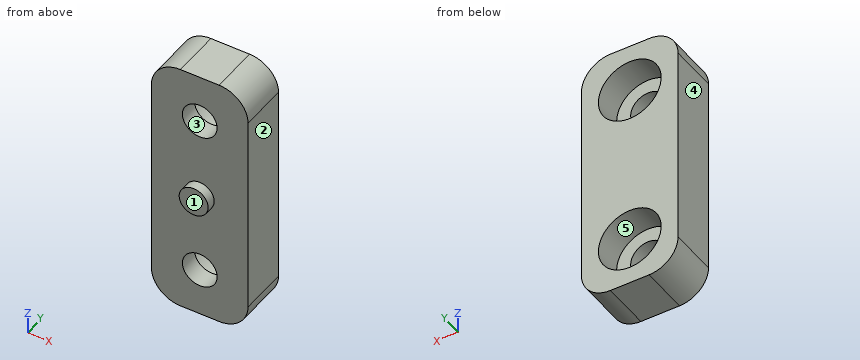
Autodesk Inventor part; units mm, degrees
ref_plane "YZ Plane" through (0, 0, 0) normal (1, 0, 0) x (0, 1, 0)
ref_plane "XZ Plane" through (0, 0, 0) normal (0, 1, 0) x (-1, 0, 0)
ref_plane "XY Plane" through (0, 0, 0) normal (0, 0, 1) x (1, 0, 0)
sketch "Sketch1" plane through (0, 0, 0) normal (0, 1, 0) x (-1, 0, 0)
  line L0 (5, -13.5) -> (-5, -13.5)
  line L1 (-5, -13.5) -> (-5, 13.5)
  line L2 (-5, 13.5) -> (5, 13.5)
  line L3 (5, 13.5) -> (5, -13.5)
  line L4 (5, -13.5) -> (-5, 13.5) construction
  line L5 (-5, -13.5) -> (5, 13.5) construction
  circle A0 centre (0, -8.5) radius 3.25
  circle A1 centre (0, 8.5) radius 3.25
  circle A2 centre (0, 0) radius 1.5
  dimension "d0" = 17
  dimension "d1" = 6.5
  dimension "d2" = 6.5
  dimension "d3" = 3
  dimension "d4" = 5
  dimension "d5" = 5
  dimension "d6" = 5
extrude "Extrusion1" add sketch "Sketch1" along normal blind 5 contours L0 L1 L2 L3 | A0 | A1 | A2
sketch "Sketch2" plane through (0, 0, 0) normal (0, -1, 0) x (1, 0, 0)
  circle A0 centre (0, 0) radius 1.5
  dimension "d9" = 3
extrude "Extrusion2" add sketch "Sketch2" along normal blind 1
sketch "Sketch3" plane through (0, 5, 0) normal (0, 1, 0) x (1, 0, 0)
  line L0 (-5, -13.5) -> (5, -13.5)
  line L1 (5, -13.5) -> (5, 13.5)
  line L2 (5, 13.5) -> (-5, 13.5)
  line L3 (-5, 13.5) -> (-5, -13.5)
  point P0 (0, 0)
  point P1 (0, 8.5)
  point P2 (0, -8.5)
  dimension "d12" = 8.5
  dimension "d13" = 8.5
hole "Hole1" at (0, 5, -8.5) at (0, 5, 8.5) direction (0, -1, 0) diameter 3.6 depth 28.25 tip angle 118 counterbore diameter 6.5 counterbore depth 3
fillet "Fillet1" radius 3 4 edges at (5, 2.5, 13.5) (5, 2.5, -13.5) (-5, 2.5, -13.5) (-5, 2.5, 13.5)
sketch "Sketch4" plane through (0, 2, -8.5) normal (0, 1, 0) x (1, 0, 0)
  circle A0 centre (0, 0) radius 1.8
  circle A1 centre (0, -17) radius 1.8
  point P0 (0, -8.5)
extrude "Extrusion3" [suppressed]
properties part number "Belt Clamp Block" material "ABS Plastic"
Design review of the part built by this model. Coordinates are the model's own, in mm. Face numbers are marked on the shaded views. A direction names the side the tool comes from. Coordinates: 2 decimals unless noted, no trailing zeros. Loops run counter-clockwise (first coordinate to the right, second up) from the corner with the lowest first, then second, coordinate; pieces in that order, holes last.
Item 1: Add section D-D (z = 5.5). Write out the cut boundary in (x, y), and give its area (3 significant figures).
Completed:
outline: (-5, 0) - (5, 0) - (5, 5) - (1.25, 5) - (1.25, 2) - (-1.25, 2) - (-1.25, 5) - (-5, 5) - close
area: 42.5 mm2
Item 2: Add section C-C (z = 8.5). Write out the cut boundary in (x, y), and give its area (3 significant figures).
Completed:
outline: (-5, 0) - (-1.8, 0) - (-1.8, 2) - (-3.25, 2) - (-3.25, 5) - (-5, 5) - close; (1.8, 0) - (5, 0) - (5, 5) - (3.25, 5) - (3.25, 2) - (1.8, 2) - close
area: 23.3 mm2
Item 3: Draft analysis for pull direction X (two halves, no side actions). For the marked faces 1, 2 and 3, state which applies: pulls with the +X half, pulls with the -X half, needs draft (parallel to the pull), parting line crosses it, or undercut.
Completed:
face 1: needs draft
face 2: pulls with the +X half
face 3: undercut
Item 4: Add section B-B (y = 4.15). Write out the cut boundary in (x, z).
Completed:
outline: (-5, -10.5) arc R3 ccw to (-2, -13.5) - (2, -13.5) arc R3 ccw to (5, -10.5) - (5, 10.5) arc R3 ccw to (2, 13.5) - (-2, 13.5) arc R3 ccw to (-5, 10.5) - close; hole circle Ø6.5 at (0, -8.5); hole circle Ø6.5 at (0, 8.5)
Item 5: Clearance check with flat-ended pins moving along their axes: pin 1 (3 mm diameter, centred on x = 0, z = 8.5, fed in from +Y); pin 2 (1.5 mm diameter, centred on x = -0.5, z = -3.5, fed in from -Y); pin 3 (3 mm diameter, centred on x = -2.5, y = 4, fed in from -Z); pin 4 (6 mm diameter, centred on x = 0, z = -8.5, fed in from +Y). State where each tip first meets the part, or that it passes through.
Completed:
pin 1: passes through
pin 2: stops at y = 0
pin 3: stops at z = -13.5
pin 4: stops at y = 2
Item 6: Add section A-A (x = 0). Write out the cut boundary in (y, z), and give its area (3 significant figures).
Completed:
outline: (-1, -1.5) - (0, -1.5) - (0, -6.7) - (2, -6.7) - (2, -5.25) - (5, -5.25) - (5, 5.25) - (2, 5.25) - (2, 6.7) - (0, 6.7) - (0, 1.5) - (-1, 1.5) - close; (0, -13.5) - (5, -13.5) - (5, -11.75) - (2, -11.75) - (2, -10.3) - (0, -10.3) - close; (0, 10.3) - (2, 10.3) - (2, 11.75) - (5, 11.75) - (5, 13.5) - (0, 13.5) - close
area: 84.6 mm2
Item 7: Wall thickness on L1, parallel to Z at x = 0, y = 3.65; L2, parallel to Z at x = 0, y = 1.15; L3, parallel to X at y = 2.85, z = 8.5: over which ranges is each line inside the solid? List them lowest first.
Completed:
L1: z = -13.5 to -11.75, -5.25 to 5.25, 11.75 to 13.5
L2: z = -13.5 to -10.3, -6.7 to 6.7, 10.3 to 13.5
L3: x = -5 to -3.25, 3.25 to 5
Item 8: For the marked faces 4 and 5, list the 3-axis set-ups (+Z, -Z, +X, -X, +Y, -Y) from which the entire face can be reached by the end or side of a thin tool; tool diameter is ignored.
Completed:
face 4: +Z, -Z, -X, +Y, -Y
face 5: +Y
